Work out the finished part from the listing and answer in its coordinate system (mm). A direction names the side the tool comes from. Give positions to 0.01 mm unless a question says otherwise; leave off trailing zeros. Order: outer loops, then holes, each group sorted by start corner. A loop starts at its lowest first (then second) coordinate and runs counter-clockwise, first axis right, second up. Notation, with made-up numbers: M 19.5,47 L 72.5,47 A11 ccw 72.5,61 Z; hole C 86.5,-9.5 d7. An arc over 180 degrees is marked long. One line per item, written item: value.
from build123d import *

# Parameters (mm, degrees)
SKIZZE1_W                       = 140
SKIZZE1_H                       = 140
SKIZZE1_W_2                     = 46
SKIZZE1_H_2                     = 46
AUFSATZ_LINEAR_AUSTRAGEN1_DEPTH = 10
SKIZZE3_W                       = 40.5
SKIZZE3_H                       = 40.5
SCHNITT_LINEAR_AUSTRAGEN1_DEPTH = 1
VERRUNDUNG1_R                   = 1


with BuildPart() as part:
    # Skizze1 → Aufsatz-Linear austragen1 (new body)
    with BuildSketch(Plane(origin=(0, 0, 0), x_dir=(1, 0, 0), z_dir=(0, 1, 0))):
        with Locations((70, 70)):
            Rectangle(SKIZZE1_W, SKIZZE1_H)
        with Locations((70, 70)):
            Rectangle(SKIZZE1_W_2, SKIZZE1_H_2, mode=Mode.SUBTRACT)
    extrude(amount=AUFSATZ_LINEAR_AUSTRAGEN1_DEPTH)

    # Skizze3 → Schnitt-Linear austragen1 (cut)
    with BuildSketch(Plane(origin=(0, 10, 0), x_dir=(1, 0, 0), z_dir=(0, 1, 0))):
        with Locations((70, 118.25)):
            Rectangle(SKIZZE3_W, SKIZZE3_H)
    extrude(amount=-SCHNITT_LINEAR_AUSTRAGEN1_DEPTH, mode=Mode.SUBTRACT)

    # Verrundung1
    verrundung1_edges = [part.edges().sort_by_distance(p)[0] for p in [
        (47, 5, -93),
        (47, 5, -47),
        (93, 5, -47),
        (93, 5, -93),
    ]]
    fillet(verrundung1_edges, radius=VERRUNDUNG1_R)


solid = part.part
(1) Section A-A, the plane z = -53 is taken. Give the vertices of the cut face in (x, y).
Findings:
outline: M 0,0 L 47,0 L 47,10 L 0,10 Z; M 93,0 L 140,0 L 140,10 L 93,10 Z
(2) Which of the six approach directions +Z, -Z, +X, -X, +Y, -Y give full straight-line access (tool end or side, diameter ignored) to faces 4 (the flat face through (70, 5, -47)), 5 (the flat face through (69, 10, -40)), 6 (the flat face through (70, 9, -119))?
Findings:
face 4: +Y, -Y
face 5: +Z, -Z, +X, -X, +Y
face 6: +Y
(3) Determine the mould class of faces 1 (the flat face through (70, 5, -93)), 2 (the flat face through (38, 0, -71)), 3 (the flat face through (0, 5, -69)) for opening direction X: pulls with the +X half, pulls with the -X half, needs draft (parallel to the pull), parting line crosses it, or undercut.
Findings:
face 1: undercut
face 2: needs draft
face 3: pulls with the -X half
(4) Section C-C, the plane y = 6.5 is taken. Give the vertices of the cut face in (x, z).
Findings:
outline: M 0,-140 L 140,-140 L 140,0 L 0,0 Z; hole M 47,-92 A1 ccw 48,-93 L 92,-93 A1 ccw 93,-92 L 93,-48 A1 ccw 92,-47 L 48,-47 A1 ccw 47,-48 Z
(5) Given P1, Ø8, axis at x = 71, z = -121, coming from the +Y side, flat-ended and moving along its own axis, determine where the tip first touches the part or whether it passes through.
Findings:
P1: stops at y = 9
(6) Section D-D, the plane z = -120 is taken. Give the vertices of the cut face in (x, y), then the cut area to 3 significant figures.
Findings:
outline: M 0,0 L 140,0 L 140,10 L 90.25,10 L 90.25,9 L 49.75,9 L 49.75,10 L 0,10 Z
area: 1,360 mm^2
(7) Section B-B, the plane x = 69 is taken. Give the vertices of the cut face in (y, z).
Findings:
outline: M 0,-140 L 10,-140 L 10,-138.5 L 9,-138.5 L 9,-98 L 10,-98 L 10,-93 L 0,-93 Z; M 0,-47 L 10,-47 L 10,0 L 0,0 Z
(8) Find the intervals of material crossed by probe 1 along Z at (x, y) = (67.5, 9.5); probe 2 along X at (y, z) = (2, -88); probe 3 along Z at (x, y) = (68.5, 6.5), in increasing order. Write a range as from..to.
Findings:
probe 1: z = -140..-138.5, -98..-93, -47..0
probe 2: x = 0..47, 93..140
probe 3: z = -140..-93, -47..0
